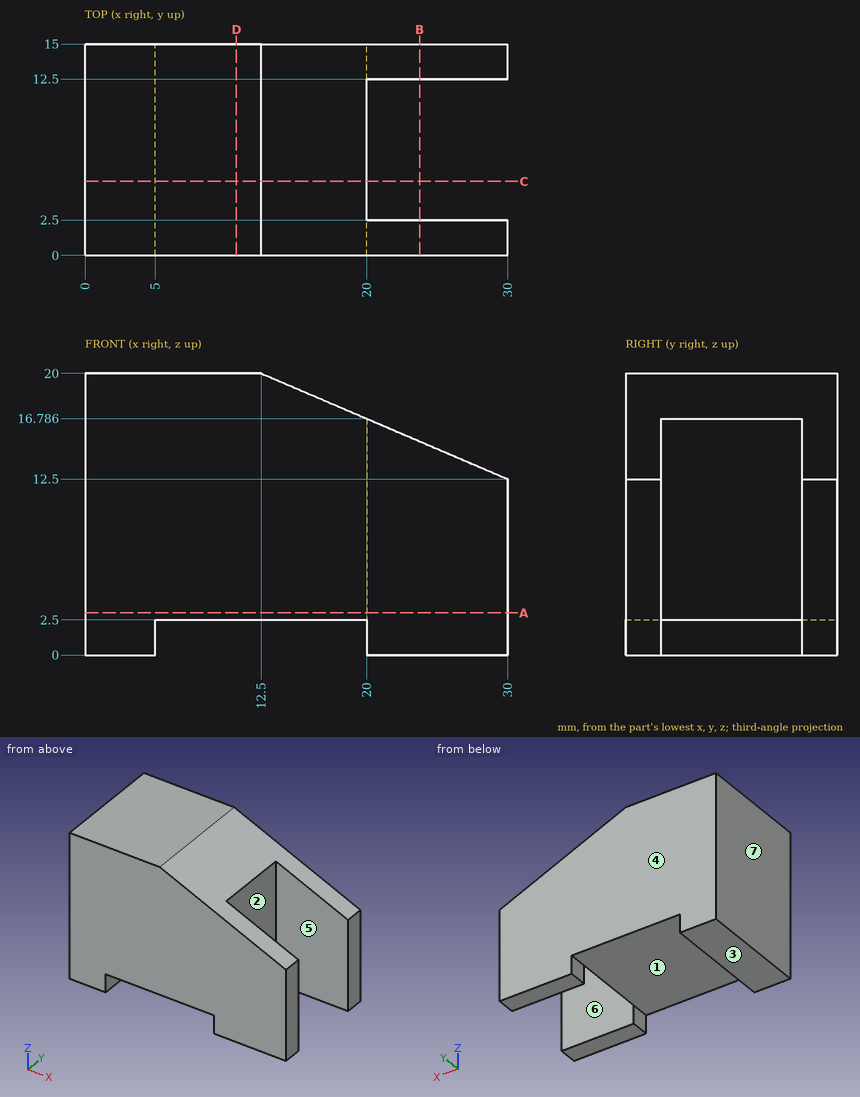
Check sheet for the drawn part. Datum: minimum x, y, z corner. Units: mm. A direction names the side the tool comes from. Coordinates: 2 decimals unless noted, no trailing zeros. Write each loop counter-clockwise with the first axis right and the second up, starting at its lowest first coordinate (ties: lowest second). Pieces come first, ordered by that corner, then holes. Notation, with made-up numbers: M -12,-25 L -5,-25 A10 ccw -5,-6 Z; hole C 10,59 d5. An arc over 180 degrees is marked long. Use a Markdown table: item, result.
Q1. Thickness scan on line 1 (Y direction, x = 24, z = 13.5); line 2 (X direction, y = 6, z = 1.5); line 3 (Z direction, x = 8.75, y = 5.5). Record the ranges inside material, lowest first.
Reply:
| item | result |
|---|---|
| line 1 | y = 0 to 2.5, 12.5 to 15 |
| line 2 | x = 0 to 5 |
| line 3 | z = 2.5 to 20 |
Q2. Sectioned sample at D-D, the plane x = 10.75. Record the boundary of the cut face in (y, z), plus the area to 4 significant figures.
Reply:
| item | result |
|---|---|
| outline | M 0,2.5 L 15,2.5 L 15,20 L 0,20 Z |
| area | 262.5 mm² |
Q3. Set-up check for the marked faces 1, 2 and 3: record each of +Z, -Z, +X, -X, +Y, -Y from which the full face is reachable in a straight line by a thin tool's end or side.
Reply:
| item | result |
|---|---|
| face 1 | -Z, +Y, -Y |
| face 2 | +Z, -Z, +X |
| face 3 | -Z, +X, -X, +Y, -Y |
Q4. Sectioned sample at B-B, the plane x = 23.75. Record the boundary of the cut face in (y, z), plus the area to 3 significant figures.
Reply:
| item | result |
|---|---|
| outline | M 0,0 L 2.5,0 L 2.5,15.18 L 0,15.18 Z; M 12.5,0 L 15,0 L 15,15.18 L 12.5,15.18 Z |
| area | 75.9 mm² |
Q5. Sectioned sample at A-A, the plane z = 3. Record the boundary of the cut face in (x, y).
Reply:
| item | result |
|---|---|
| outline | M 0,0 L 30,0 L 30,2.5 L 20,2.5 L 20,12.5 L 30,12.5 L 30,15 L 0,15 Z |
Q6. Draft check along Y on the marked faces 4, 5, 6 and 7. Enter one of: +Y half, -Y half, draft (parallel to the pull), parting line (faces both ways), or undercut.
Reply:
| item | result |
|---|---|
| face 4 | +Y half |
| face 5 | undercut |
| face 6 | undercut |
| face 7 | draft |
Q7. Sectioned sample at C-C, the plane y = 5.25. Record the boundary of the cut face in (x, z), plus the area to 3 significant figures.
Reply:
| item | result |
|---|---|
| outline | M 0,0 L 5,0 L 5,2.5 L 20,2.5 L 20,16.79 L 12.5,20 L 0,20 Z |
| area | 350 mm² |
Q8. Go/stop test with flat-tipped pins: P1, Ø2, axis at y = 6.5, z = 1, coming from the +X side; P2, Ø2, axis at x = 18.5, y = 12.5, coming from the +Z side; P3, Ø6, axis at x = 20.5, y = 8, coming from the -Z side. Record where each tip stops, or that it passes through.
Reply:
| item | result |
|---|---|
| P1 | stops at x = 5 |
| P2 | stops at z = 17.86 |
| P3 | stops at z = 2.5 |
